Model file for the job. Use its own axes, mm. Round coordinates to 2 decimals unless told otherwise and drop trailing zeros. Loops run counter-clockwise (first coordinate to the right, second up) from the corner with the lowest first, then second, coordinate; pieces in that order, holes last. Notation, with made-up numbers: M 43.5,50 L 64.5,50 A17 ccw 64.5,80 Z; hole C 28.5,-4.5 d2. An arc over 180 degrees is marked long. Use a Markdown table: item, result. Add a question column.
Q1. Probe line 1 (Y direction, x = -43.5, z = 22); line 2 (Y direction, x = -37, z = 4.5); line 3 (X direction, y = 2, z = 18). List the from-to ranges inside material, lowest first. Write a range as from..to.
Q2. Cut at B-B (x = -26.5). Give the cut face in (y, z).
Q3. Pin check, flat tips, straight feed: pin 1 (5 mm diameter, centred on y = -0.5, z = 6.5, fed in from +X); pin 2 (6 mm diameter, centred on y = -2, z = 27, fed in from -X). Stop position of each tip, or through.
Q4. Cut at A-A (z = 23). Give the cut face in (x, y).
from build123d import *

# Parameters (mm, degrees)
SALIENTE_EXTRUIR1_DEPTH = 32
CORTAR_EXTRUIR1_DEPTH   = 33
CROQUIS4_R              = 1
SALIENTE_EXTRUIR2_DEPTH = 0.005


with BuildPart() as part:
    # Croquis1 → Saliente-Extruir1 (new body)
    with BuildSketch(Plane.XY):
        Polygon((-51.959662641, 14.148169014), (-51.959662641, 3.148169014), (-35.959662641, -4.290206314), (-19.959662641, 3.148169014), (-19.959662641, 14.148169014), align=None)
    extrude(amount=SALIENTE_EXTRUIR1_DEPTH)

    # Croquis2 → Cortar-Extruir1 (cut)
    with BuildSketch(Plane(origin=(-19.959662641, 0, 0), x_dir=(0, 0, -1), z_dir=(1, 0, 0))):
        Polygon((0, -4.290206314), (-16, -4.290206314), (0, 3.148169014), align=None)
        Polygon((-32, -4.290206314), (-32, 3.148169014), (-16, -4.290206314), align=None)
    extrude(amount=-CORTAR_EXTRUIR1_DEPTH, mode=Mode.SUBTRACT)

    # Croquis4 → Saliente-Extruir2 (add)
    with BuildSketch(Plane(origin=(-4.750700642, 10.218791996, 0), x_dir=(-0.906796627, -0.421568354, 0), z_dir=(0.421568354, -0.906796627, 0))):
        with Locations((20.772186335, -16)):
            Circle(CROQUIS4_R)
    extrude(amount=SALIENTE_EXTRUIR2_DEPTH)


solid = part.part
Checked values:
| question | item | result |
|---|---|---|
| 1 | line 1 | y = -0.78..14.15 |
| 1 | line 2 | y = 1.06..14.15 |
| 1 | line 3 | x = -49.49..-22.43 |
| 2 | outline | M 0.11,6.54 L 3.15,0 L 14.15,0 L 14.15,32 L 3.15,32 L 0.11,25.46 Z |
| 3 | pin 1 | stops at x = -22.43 |
| 3 | pin 2 | stops at x = -47.34 |
| 4 | outline | M -51.96,3.15 L -42.96,-1.04 L -28.96,-1.04 L -19.96,3.15 L -19.96,14.15 L -51.96,14.15 Z |
